Read the model definition and answer for the solid it produces. Units are mm, in the model's axes. Face numbers are marked on the shaded views. A direction names the side the tool comes from. Give positions to 0.01 mm unless a question says otherwise; leave off trailing zeros. Order: outer loops, then holes, each group sorted by start corner. A loop starts at its lowest first (then second) coordinate and runs counter-clockwise, first axis right, second up.
```python
from build123d import *

# Parameters (mm, degrees)
SKETCH1_W                = 56.4
SKETCH1_H                = 56.4
BOSS_EXTRUDE1_DEPTH      = 56
SKETCH2_R                = 19.05
BOSS_EXTRUDE2_DEPTH      = 1.6
SKETCH3_R                = 3.175
BOSS_EXTRUDE3_DEPTH      = 19.4
CUT_EXTRUDE1_START       = -16
CUT_EXTRUDE1_DEPTH       = 16
F_5_0_5_DIAMETER_HOLE1_D = 5
SKETCH8_W                = 9.26
SKETCH8_H                = 9.26
CUT_EXTRUDE2_DEPTH       = 51
FILLET1_R                = 4.63


with BuildPart() as part:
    # Sketch1 → Boss-Extrude1 (new body)
    with BuildSketch(Plane(origin=(0, 0, 0), x_dir=(1, 0, 0), z_dir=(0, 1, 0))):
        Rectangle(SKETCH1_W, SKETCH1_H)
    extrude(amount=BOSS_EXTRUDE1_DEPTH)

    # Sketch2 → Boss-Extrude2 (add)
    with BuildSketch(Plane(origin=(0, 0, 0), x_dir=(1, 0, 0), z_dir=(0, 1, 0))):
        with Locations(Location((0, 0, 0), (0, 0, 270))):
            Circle(SKETCH2_R)
    extrude(amount=-BOSS_EXTRUDE2_DEPTH)

    # Sketch3 → Boss-Extrude3 (add)
    with BuildSketch(Plane.XZ.offset(1.6)):
        with Locations(Location((0, 0, 0), (0, 0, 90))):
            Circle(SKETCH3_R)
    extrude(amount=BOSS_EXTRUDE3_DEPTH)

    # Sketch4 → Cut-Extrude1 (cut)
    with BuildSketch(Plane.XZ.offset(21).offset(CUT_EXTRUDE1_START)):
        with BuildLine():
            Line((-1.78605711, 2.625), (1.78605711, 2.625))
            ThreePointArc((1.78605711, 2.625), (0, 3.175), (-1.78605711, 2.625))
        make_face()
    extrude(amount=CUT_EXTRUDE1_DEPTH, mode=Mode.SUBTRACT)

    # Ø5.0 (5) Diameter Hole1 (through all)
    with Locations(Plane(origin=(0, 0, 0), x_dir=(-1, 0, 0), z_dir=(0, -1, 0))):
        with Locations((-23.57, 23.569999995), (23.57, 23.57), (23.570000005, -23.57), (-23.569999995, -23.570000005)):
            Hole(F_5_0_5_DIAMETER_HOLE1_D / 2)

    # Sketch8 → Cut-Extrude2 (cut)
    with BuildSketch(Plane(origin=(0, 56, 0), x_dir=(1, 0, 0), z_dir=(0, 1, 0))):
        with Locations((-23.57, 23.57)):
            Rectangle(SKETCH8_W, SKETCH8_H)
        with Locations((23.57, 23.57)):
            Rectangle(SKETCH8_W, SKETCH8_H)
        with Locations((23.57, -23.57)):
            Rectangle(SKETCH8_W, SKETCH8_H)
        with Locations((-23.57, -23.57)):
            Rectangle(SKETCH8_W, SKETCH8_H)
    extrude(amount=-CUT_EXTRUDE2_DEPTH, mode=Mode.SUBTRACT)

    # Fillet1
    fillet1_edges = [part.edges().sort_by_distance(p)[0] for p in [
        (28.2, 2.5, 28.2),
        (28.2, 2.5, -28.2),
        (18.94, 30.5, -28.2),
        (28.2, 30.5, -18.94),
        (18.94, 30.5, -18.94),
        (18.94, 30.5, 18.94),
        (18.94, 30.5, 28.2),
        (28.2, 30.5, 18.94),
        (-18.94, 30.5, 18.94),
        (-18.94, 30.5, 28.2),
        (-28.2, 2.5, 28.2),
        (-28.2, 30.5, 18.94),
        (-18.94, 30.5, -28.2),
        (-28.2, 30.5, -18.94),
        (-28.2, 2.5, -28.2),
        (-18.94, 30.5, -18.94),
    ]]
    fillet(fillet1_edges, radius=FILLET1_R - 0.0001)  # a hair under: the kernel refuses the full size


solid = part.part
```
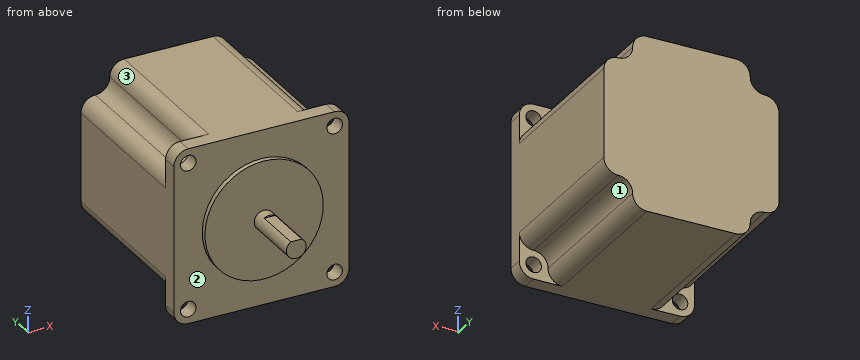
1) Consider L1, parallel to Z at x = -23.57, y = 1.45; L2, parallel to X at y = 1, z = 23. Determine where each line is inside the solid, lowest interval first.
Final values:
L1: z = -28.2 to -26.07, -21.07 to 21.07, 26.07 to 28.2
L2: x = -28.2 to -26, -21.14 to 21.14, 26 to 28.2
2) The part is cut by section A-A on z = 0. Determine the outline of the cut face in (x, y) (3 decimals), and give its area (3 significant figures).
Final values:
outline: (-28.2, 0) - (-19.05, 0) - (-19.05, -1.6) - (-3.175, -1.6) - (-3.175, -21) - (3.175, -21) - (3.175, -1.6) - (19.05, -1.6) - (19.05, 0) - (28.2, 0) - (28.2, 56) - (-28.2, 56) - close
area: 3,340 mm2
3) The part is cut by section D-D on z = 11.5. Determine the outline of the cut face in (x, y), and give its area (3 significant figures).
Final values:
outline: (-28.2, 0) - (-15.19, 0) - (-15.19, -1.6) - (15.19, -1.6) - (15.19, 0) - (28.2, 0) - (28.2, 56) - (-28.2, 56) - close
area: 3,210 mm2
4) The part is cut by section C-C on x = 0. Determine the outline of the cut face in (y, z) (3 decimals), and give its area (3 significant figures).
Final values:
outline: (-21, -3.175) - (-1.6, -3.175) - (-1.6, -19.05) - (0, -19.05) - (0, -28.2) - (56, -28.2) - (56, 28.2) - (0, 28.2) - (0, 19.05) - (-1.6, 19.05) - (-1.6, 3.175) - (-5, 3.175) - (-5, 2.625) - (-21, 2.625) - close
area: 3,330 mm2
5) Given pin 1 (6 mm diameter, centred on x = 23.57, z = -23.57, fed in from -Y); pin 2 (5 mm diameter, centred on x = -19, z = -10, fed in from -Y); pin 3 (3 mm diameter, centred on x = 1, y = -9.5, fed in from +Z) (3 decimals), each flat-ended and moving along its own axis, determine where each tip first touches the part or whether it passes through.
Final values:
pin 1: stops at y = 0
pin 2: stops at y = -1.6
pin 3: stops at z = 2.625
6) A tool of negligible diameter and unlimited length cuts with its end or side. For the marked faces 1, 2 and 3, from which of +Z, -Z, +X, -X, +Y, -Y can it reach the whole face along a straight path? Write none if from no direction.
Final values:
face 1: -Z, +X, +Y
face 2: -Y
face 3: +Z, -X, +Y
